Here's how the part is built. I have some questions about the finished solid (model axes, mm). A direction names the side the tool comes from. Coordinates: 2 decimals unless noted, no trailing zeros. Write each loop counter-clockwise with the first axis right and the second up, starting at its lowest first coordinate (ties: lowest second). Pieces come first, ordered by that corner, then holes. Notation, with made-up numbers: (-12.5, 82) -> (33.5, 82) arc R26 cw to (33.5, 109) -> close; hole circle Ø8 at (52, -10.5). An arc over 180 degrees is marked (long way). Use a Markdown table: item, result. Add a question column.
Item 1: If we mould it in two halves opening along X, with no side actions, what happens to faces 1 (the flat face through (99, -30.022, 3)), 2 (the flat face through (109.205, -33, 3)), 3 (the flat face through (-34.4, -25.14, 1.63)), 4 (the flat face through (99, -36.372, 3))? For each: pulls with the +X half, pulls with the -X half, needs draft (parallel to the pull), parting line crosses it, or undercut.
Item 2: If I drill on line 1 along Z through (x, y) = (67, -24.75); line 2 along Y through (x, z) = (-0.5, 1); line 3 along Z through (x, y) = (60, -42), over which ranges is the centre line in solid material (lowest first)? Write a range as from..to.
Item 3: On a 3-axis mill with a long thin cutter (end or side, diameter ignored), from which of +Z, -Z, +X, -X, +Y, -Y can I reach the whole of each face in a straight line? I mean faces 5 (the flat face through (-34.405, -41.284, 1.63)), 6 (the flat face through (96.334, -34.763, 3.219)). Say none if no direction works.
Item 4: Imagine slicing it at A-A, the plane z = 3. Write out the boundary of the cut face in (x, y), and give its area (3 significant figures).
```python
from build123d import *

# Parameters (mm, degrees)
F0_W      = 11.3603360951
F0_H      = 3.4401938319
F1_DEPTH  = 6.35
F2_DEPTH  = 15.61084
F3_DEPTH  = 141.03858
F4_R      = 7.62
F5_R      = 7.62
F6_SIZE2  = 5.1044321158
F6_SIZE   = 19.05
F7_SIZE2  = 14.2191135768
F7_SIZE   = 3.81
F8_SIZE2  = 14.2191135768
F8_SIZE   = 3.81
F9_R      = 1.27
F10_R     = 1.27
F13_DEPTH = 25.4
F14_SIZE  = 0.762
F15_SIZE  = 0.762


with BuildPart() as f1:
    # F0 (on Top) → F1 (new body)
    with BuildSketch(Plane.XY):
        with Locations((-37.5133920461, -25.4080276936)):
            Rectangle(F0_W, F0_H)
    extrude(amount=F1_DEPTH)

    # F2 (add): a face of the model
    f2_faces = [f1.faces().sort_by_distance(p)[0] for p in [
        (-37.5133920461, -27.1281246096, 3.175),
    ]]
    extrude(f2_faces, amount=F2_DEPTH)

    # F3 (add): a face of the model
    f3_faces = [f1.faces().sort_by_distance(p)[0] for p in [
        (-31.8332239985, -33.2134476936, 3.175),
    ]]
    extrude(f3_faces, amount=F3_DEPTH)

    # F4
    f4_edges = [f1.edges().sort_by_distance(p)[0] for p in [
        (109.205356, -42.738965, 3.175),
    ]]
    fillet(f4_edges, radius=F4_R)

    # F5
    f5_edges = [f1.edges().sort_by_distance(p)[0] for p in [
        (109.205356, -23.687931, 3.175),
    ]]
    fillet(f5_edges, radius=F5_R)

    # F6
    f6_edges = [f1.edges().sort_by_distance(p)[0] for p in [
        (-43.19356, -33.213448, 6.35),
    ]]
    chamfer(f6_edges, length=F6_SIZE, length2=F6_SIZE2)

    # F7
    f7_edges = [f1.edges().sort_by_distance(p)[0] for p in [
        (-43.19356, -23.687931, 0.622784),
    ]]
    f7_side = f1.faces().sort_by_distance((-43.19356, -33.213448, 0.622784))[0]
    chamfer(f7_edges, length=F7_SIZE, length2=F7_SIZE2, reference=f7_side)

    # F8
    f8_edges = [f1.edges().sort_by_distance(p)[0] for p in [
        (-43.19356, -42.738965, 0.622784),
    ]]
    chamfer(f8_edges, length=F8_SIZE, length2=F8_SIZE2)

    # F9
    f9_edges = [f1.edges().sort_by_distance(p)[0] for p in [
        (38.720898, -42.738965, 6.35),
    ]]
    fillet(f9_edges, radius=F9_R)

    # F10
    f10_edges = [f1.edges().sort_by_distance(p)[0] for p in [
        (36.305455, -42.738965, 0),
    ]]
    fillet(f10_edges, radius=F10_R)

    # F12 (on face) → F13 (cut)
    with BuildSketch(Plane.XY.offset(6.35)):
        Polygon((99.096596241, -36.3724566996), (100.9298735347, -36.3724566996), (102.7631508283, -33.1971272826), (100.9298735347, -30.0217978656), (97.2633189473, -30.0217978656), (95.4300416537, -33.1971272826), (97.2633189473, -36.3724566996), align=None)
    extrude(amount=-F13_DEPTH, mode=Mode.SUBTRACT)

    # F14
    f14_edges = [f1.edges().sort_by_distance(p)[0] for p in [
        (-36.084003, -40.833965, 3.150568),
    ]]
    chamfer(f14_edges, length=F14_SIZE)

    # F15
    f15_edges = [f1.edges().sort_by_distance(p)[0] for p in [
        (-36.084003, -25.592931, 3.150568),
    ]]
    chamfer(f15_edges, length=F15_SIZE)


solid = f1.part
```
Ans:
| question | item | result |
|---|---|---|
| 1 | face 1 | undercut |
| 1 | face 2 | pulls with the +X half |
| 1 | face 3 | pulls with the -X half |
| 1 | face 4 | undercut |
| 2 | line 1 | z = 0.02..6.33 |
| 2 | line 2 | y = -42.71..-23.72 |
| 2 | line 3 | z = 0.12..6.23 |
| 3 | face 5 | +Z, -Z, -X, -Y |
| 3 | face 6 | +Z, -Z |
| 4 | outline | (-36.65, -39.9) -> (-33.71, -41.47) -> (-28.97, -42.74) -> (101.59, -42.74) arc R7.62 ccw to (109.21, -35.12) -> (109.21, -31.31) arc R7.62 ccw to (101.59, -23.69) -> (-28.97, -23.69) -> (-33.71, -24.96) -> (-36.65, -26.53) -> close; hole (95.43, -33.2) -> (97.26, -36.37) -> (100.93, -36.37) -> (102.76, -33.2) -> (100.93, -30.02) -> (97.26, -30.02) -> close |
| 4 | area | 2,700 mm^2 |
